from build123d import *

# Parameters (mm, degrees)
F1_DEPTH = 60
F3_D     = 5
F4_W     = 35
F4_H     = 20
F5_DEPTH = 25
F6_R     = 5


with BuildPart() as f1:
    # F0 (on Top) → F1 (new body)
    with BuildSketch(Plane.XY):
        Polygon((0, 69), (0, 0), (6, 0), (6, 63), (59, 63), (59, 0), (65, 0), (65, 69), align=None)
    extrude(amount=F1_DEPTH)

    # F3 (through all)
    with Locations(Plane(origin=(0, 69, 0), x_dir=(-1, 0, 0), z_dir=(0, 1, 0))):
        with Locations((-32.5, 30)):
            Hole(F3_D / 2)

    # F4 (on face) → F5 (cut)
    with BuildSketch(Plane(origin=(0, 69, 0), x_dir=(-1, 0, 0), z_dir=(0, 1, 0))):
        with Locations((-32.5, 50)):
            Rectangle(F4_W, F4_H)
    extrude(amount=-F5_DEPTH, mode=Mode.SUBTRACT)

    # F6
    f6_edges = [f1.edges().sort_by_distance(p)[0] for p in [
        (15, 66, 60),
        (50, 66, 60),
    ]]
    fillet(f6_edges, radius=F6_R)


solid = f1.part
Input: part model. Units: mm. Frame: model coordinates. A direction names the side the tool comes from. Give positions to 0.01 mm unless a question says otherwise; leave off trailing zeros. Loops run counter-clockwise (first coordinate to the right, second up) from the corner with the lowest first, then second, coordinate; pieces in that order, holes last. Notation, with made-up numbers: (6.5, -32) -> (44.5, -32) arc R15 ccw to (44.5, -13) -> close; hole circle Ø9 at (80, 13.5). An arc over 180 degrees is marked (long way). Answer as a JSON object with one key per item and string values. Group by question number.
Item 1: Pin query (flat end, axial travel): P1, Ø10, axis at x = 42.5, z = 23.5, coming from the -Y side; P2, Ø18, axis at y = 32, z = 18.5, coming from the -X side; P3, Ø3, axis at x = 29.5, y = 65, coming from the +Z side. Return the tip coordinate at first contact, or that it passes through.
Item 2: Cut plane A-A, the plane x = 32.5. Return the cut outline in (y, z), and give its area (3 significant figures).
Item 3: Line query: probe 1 along X at (y, z) = (8, 27.5); probe 2 along Z at (x, y) = (32.5, 66.8); probe 3 along Y at (x, z) = (17, 25). Output: solid intervals per line, ascending.
Item 4: Cut plane D-D, the plane z = 44. Return the cut outline in (x, y).
Item 5: Pull-direction query (X, two-part tool) for faces 1 (the flat face through (3, 0, 30)), 2 (the flat face through (0, 35, 30)), 3 (the flat face through (6, 31, 30)), 4 (the cylindrical face through (34, 66, 32)); classes: released by +X, released by -X, zero draft, split by the parting line, or undercut.
Item 6: Reachability of faces 5 (the flat face through (62, 35, 60)), 6 (the flat face through (32, 63, 23)), 7 (the flat face through (50, 66, 47)) from +Z, -Z, +X, -X, +Y, -Y: full face, straight path, thin tool, end or side. Return the list, or none.
Item 7: Cut plane B-B, the plane z = 30. Return the cut outline in (x, y), and give its area (3 significant figures).
Item 8: Cut plane C-C, the plane y = 39. Return the cut outline in (x, z).
Checks:
{
 "1": {"P1": "stops at y = 63", "P2": "stops at x = 0", "P3": "stops at z = 40"},
 "2": {"outline": "(63, 0) -> (69, 0) -> (69, 27.5) -> (63, 27.5) -> close; (63, 32.5) -> (69, 32.5) -> (69, 40) -> (63, 40) -> close", "area": "210 mm²"},
 "3": {"probe 1": "x = 0 to 6, 59 to 65", "probe 2": "z = 0 to 27.5, 32.5 to 40", "probe 3": "y = 63 to 69"},
 "4": {"outline": "(0, 0) -> (6, 0) -> (6, 63) -> (15, 63) -> (15, 69) -> (0, 69) -> close; (50, 63) -> (59, 63) -> (59, 0) -> (65, 0) -> (65, 69) -> (50, 69) -> close"},
 "5": {"face 1": "zero draft", "face 2": "released by -X", "face 3": "undercut", "face 4": "undercut"},
 "6": {"face 5": "+Z, +X, -X, +Y, -Y", "face 6": "+Z, -Z, -Y", "face 7": "+Z, +Y, -Y"},
 "7": {"outline": "(0, 0) -> (6, 0) -> (6, 63) -> (30, 63) -> (30, 69) -> (0, 69) -> close; (35, 63) -> (59, 63) -> (59, 0) -> (65, 0) -> (65, 69) -> (35, 69) -> close", "area": "1,120 mm²"},
 "8": {"outline": "(0, 0) -> (6, 0) -> (6, 60) -> (0, 60) -> close; (59, 0) -> (65, 0) -> (65, 60) -> (59, 60) -> close"}
}
